The listing builds one solid part. Answer for the finished solid, in the listing's coordinates (mm). Face numbers are marked on the shaded views. Give positions to 0.01 mm unless a question says otherwise; leave off trailing zeros. Loops run counter-clockwise (first coordinate to the right, second up) from the corner with the lowest first, then second, coordinate; pieces in that order, holes last. Notation, with made-up numbers: (88.25, -29) - (127.25, -29) arc R16 ccw to (127.25, -3) - close; hole circle Ø3 at (42.5, 28). An arc over 180 degrees is marked (long way). Write each question's results on one line, items separated by ' | '.
Autodesk Inventor part; units mm, degrees
ref_plane "YZ Plane" through (0, 0, 0) normal (1, 0, 0) x (0, 1, 0)
ref_plane "XZ Plane" through (0, 0, 0) normal (0, 1, 0) x (-1, 0, 0)
ref_plane "XY Plane" through (0, 0, 0) normal (0, 0, 1) x (1, 0, 0)
sketch "Sketch1" plane through (0, 0, 0) normal (0, 1, 0) x (-1, 0, 0)
  line L0 (0, 30) -> (66, 30) construction
  line L1 (66, 36.5) -> (60, 36.5)
  line L2 (60, 36.5) -> (60, 48.5) construction
  line L3 (60, 48.5) -> (66, 48.5)
  line L4 (66, 48.5) -> (66, 36.5)
  line L5 (60, 48.5) -> (60, 60)
  line L6 (60, 60) -> (6, 60)
  line L7 (66, 23.5) -> (60, 23.5)
  line L8 (60, 23.5) -> (60, 11.5) construction
  line L9 (60, 11.5) -> (66, 11.5)
  line L10 (66, 11.5) -> (66, 23.5)
  line L11 (60, 11.5) -> (60, 0)
  line L12 (60, 36.5) -> (60, 23.5)
  line L13 (33, 30) -> (33, 0) construction
  line L14 (0, 36.5) -> (6, 36.5)
  line L15 (6, 36.5) -> (6, 48.5) construction
  line L16 (6, 48.5) -> (0, 48.5)
  line L17 (0, 48.5) -> (0, 36.5)
  line L18 (6, 48.5) -> (6, 60)
  line L19 (0, 23.5) -> (6, 23.5)
  line L20 (6, 23.5) -> (6, 11.5) construction
  line L21 (6, 11.5) -> (0, 11.5)
  line L22 (0, 11.5) -> (0, 23.5)
  line L23 (6, 11.5) -> (6, 0)
  line L24 (6, 36.5) -> (6, 23.5)
  line L25 (6, 0) -> (60, 0)
  dimension "d2" = 6
  dimension "d3" = 12
  dimension "d4" = 18.5
  dimension "d5" = 33
  dimension "d6" = 11.5
  dimension "d7" = 0
extrude "Extrusion1" add sketch "Sketch1" along normal blind 6
sketch "Sketch2" plane through (0, 6, 0) normal (0, 1, 0) x (1, 0, 0)
  line L0 (-6, -36.5) -> (-6, -23.5)
  line L1 (-6, -30) -> (-60, -30) construction
  line L2 (-60, -23.5) -> (-60, -36.5)
  line L3 (-6, 0) -> (-60, 0)
  line L4 (-33, 0) -> (-33, -60) construction
  line L5 (-6, -60) -> (-60, -60)
  circle A0 centre (-49, -46) radius 4.5
  circle A1 centre (-17, -14) radius 4.5
  circle A2 centre (-33, -30) radius 4.5
  circle A3 centre (-14, -30) radius 1
  circle A4 centre (-52, -30) radius 1
  point P0 (0, 0)
  dimension "d16" = 9
  dimension "d17" = 9
  dimension "d18" = 16
  dimension "d19" = 16
  dimension "d20" = 16
  dimension "d21" = 16
  dimension "d22" = 9
  dimension "d23" = 2
  dimension "d24" = 2
  dimension "d25" = 19
  dimension "d26" = 19
extrude "Extrusion2" cut sketch "Sketch2" against normal through all
properties part number "thumper-bumper-top-v2"
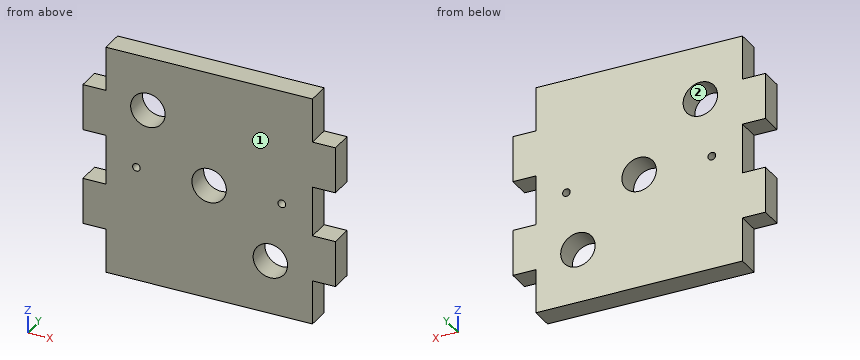
Item 1: For a pull along X with two mould halves and no side action, classify the marked faces 1 and 2 as released by +X, released by -X, zero draft, split by the parting line, or undercut.
Values found:
face 1: zero draft | face 2: undercut
Item 2: Find the intervals of material crossed by line 1 along X through (y, z) = (3.95, 30); line 2 along X through (y, z) = (1.7, 46); line 3 along Z through (x, y) = (-33, 4.2), in increasing order. Write a range as [from, to].
Values found:
line 1: x = [-60, -53], [-51, -37.5], [-28.5, -15], [-13, -6] | line 2: x = [-66, -53.5], [-44.5, 0] | line 3: z = [0, 25.5], [34.5, 60]
Item 3: A cutting plane is placed at C-C, the plane y = 2.45. Determine the outline of the cut face in (x, z).
Values found:
outline: (-66, 11.5) - (-60, 11.5) - (-60, 0) - (-6, 0) - (-6, 11.5) - (0, 11.5) - (0, 23.5) - (-6, 23.5) - (-6, 36.5) - (0, 36.5) - (0, 48.5) - (-6, 48.5) - (-6, 60) - (-60, 60) - (-60, 48.5) - (-66, 48.5) - (-66, 36.5) - (-60, 36.5) - (-60, 23.5) - (-66, 23.5) - close; hole circle Ø9 at (-49, 46); hole circle Ø2 at (-52, 30); hole circle Ø9 at (-33, 30); hole circle Ø9 at (-17, 14); hole circle Ø2 at (-14, 30)
Item 4: A cutting plane is placed at D-D, the plane z = 52.5. Determine the outline of the cut face in (x, y).
Values found:
outline: (-60, 0) - (-6, 0) - (-6, 6) - (-60, 6) - close
Item 5: A cutting plane is placed at B-B, the plane x = -17. Determine the outline of the cut face in (y, z), plus the area to 3 significant figures.
Values found:
outline: (0, 0) - (6, 0) - (6, 9.5) - (0, 9.5) - close; (0, 18.5) - (6, 18.5) - (6, 60) - (0, 60) - close | area: 306 mm²
Item 6: A cutting plane is placed at A-A, the plane z = 14. Determine the outline of the cut face in (x, y), plus the area to 3 significant figures.
Values found:
outline: (-66, 0) - (-21.5, 0) - (-21.5, 6) - (-66, 6) - close; (-12.5, 0) - (0, 0) - (0, 6) - (-12.5, 6) - close | area: 342 mm²
Item 7: Flat-ended cylindrical pins translate along their axes: P1, Ø1.8, axis at y = 3.5, z = 5, coming from the +X side; P2, Ø8, axis at x = -49, z = 46, coming from the +Y side; P3, Ø3, axis at y = 3, z = 6.5, coming from the -X side. Find the tip coordinate at first contact, or state that the pin passes through.
Values found:
P1: stops at x = -6 | P2: passes through | P3: stops at x = -60
